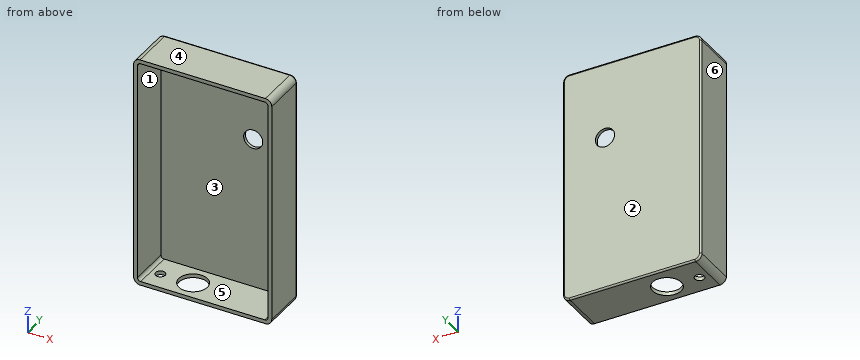
Autodesk Inventor part; units mm, degrees
ref_plane "YZ Plane" through (0, 0, 0) normal (1, 0, 0) x (0, 1, 0)
ref_plane "XZ Plane" through (0, 0, 0) normal (0, 1, 0) x (-1, 0, 0)
ref_plane "XY Plane" through (0, 0, 0) normal (0, 0, 1) x (1, 0, 0)
sketch "Skizze1" plane through (0, 0, 0) normal (0, 1, 0) x (-1, 0, 0)
  line L0 (1, 0) -> (40, 0)
  line L1 (41, 1) -> (41, 70)
  line L2 (40, 71) -> (1, 71)
  line L3 (0, 70) -> (0, 1)
  line L4 (42.2, 70.2) -> (42.2, 0.8)
  line L5 (40.2, -1.2) -> (0.8, -1.2)
  line L6 (-1.2, 0.8) -> (-1.2, 70.2)
  line L7 (0.8, 72.2) -> (40.2, 72.2)
  arc A0 (42.2, 70.2) -> (40.2, 72.2) centre (40.2, 70.2) ccw
  arc A1 (40.2, -1.2) -> (42.2, 0.8) centre (40.2, 0.8) ccw
  arc A2 (-1.2, 0.8) -> (0.8, -1.2) centre (0.8, 0.8) ccw
  arc A3 (0.8, 72.2) -> (-1.2, 70.2) centre (0.8, 70.2) ccw
  arc A4 (41, 70) -> (40, 71) centre (40, 70) ccw
  arc A5 (40, 0) -> (41, 1) centre (40, 1) ccw
  arc A6 (0, 1) -> (1, 0) centre (1, 1) ccw
  arc A7 (1, 71) -> (0, 70) centre (1, 70) ccw
  point P0 (0, 0)
  point P1 (41, 71)
  point P2 (41, 0)
  point P3 (0, 71)
  dimension "d0" = 41
  dimension "d1" = 71
  dimension "d2" = 1.2
  dimension "d3" = 2
  dimension "d4" = 1
extrude "Extrusion1" add sketch "Skizze1" along normal blind 13
sketch "Skizze2" plane through (0, 13, 0) normal (0, 1, 0) x (1, 0, 0)
  line L0 (1.2, -70.2) -> (1.2, -0.8)
  arc A0 (1.2, -0.8) -> (-0.8, 1.2) centre (-0.8, -0.8) ccw
  line L1 (-0.8, 1.2) -> (-40.2, 1.2)
  arc A1 (-40.2, 1.2) -> (-42.2, -0.8) centre (-40.2, -0.8) ccw
  line L2 (-42.2, -0.8) -> (-42.2, -70.2)
  arc A2 (-42.2, -70.2) -> (-40.2, -72.2) centre (-40.2, -70.2) ccw
  line L3 (-40.2, -72.2) -> (-0.8, -72.2)
  arc A3 (-0.8, -72.2) -> (1.2, -70.2) centre (-0.8, -70.2) ccw
  arc A4 (0, -1) -> (-1, 0) centre (-1, -1) ccw
  line L4 (0, -1) -> (0, -70)
  arc A5 (-1, -71) -> (0, -70) centre (-1, -70) ccw
  line L5 (-1, -71) -> (-40, -71)
  arc A6 (-41, -70) -> (-40, -71) centre (-40, -70) ccw
  line L6 (-41, -70) -> (-41, -1)
  arc A7 (-40, 0) -> (-41, -1) centre (-40, -1) ccw
  line L7 (-40, 0) -> (-1, 0)
  point P0 (0, 0)
extrude "Extrusion2" add sketch "Skizze2" along normal blind 1 contours A3 L3 A2 L2 A1 L1 A0 L0 | L4 A5 L5 A6 L6 A7 L7 A4
fillet "Rundung1" radius 0.5 8 edges at (0.6142, 14, -0.6142) (-20.5, 14, -1.2) (-41.6142, 14, -0.6142) (-42.2, 14, 35.5) (-41.6142, 14, 71.6142) (-20.5, 14, 72.2) (0.6142, 14, 71.6142) (1.2, 14, 35.5)
sketch "Skizze3" plane through (0, 14, 0) normal (0, 1, 0) x (1, 0, 0)
  circle A0 centre (-12, -48) radius 3
  line L0 (0, -1) -> (0, -70)
  line L1 (-40, 0) -> (-1, 0)
  point P0 (0, 0)
  dimension "d10" = 6
  dimension "d11" = 12
  dimension "d12" = 48
extrude "Extrusion3" cut sketch "Skizze3" against normal blind 1
sketch "Skizze4" plane through (-0.8, 0, -1.2) normal (0, 0, -1) x (-1, 0, 0)
  circle A0 centre (26.4, 6.5) radius 4.5
  line L0 (0, 0) -> (39.4, 0)
  line L1 (41.4, 0) -> (41.4, 13.5)
  circle A1 centre (36.4, 6) radius 1.5
  point P0 (-0.8, 0)
  dimension "d15" = 9
  dimension "d16" = 6.5
  dimension "d17" = 15
  dimension "d18" = 3
  dimension "d19" = 5
extrude "Extrusion4" cut sketch "Skizze4" against normal blind 5
properties part number "wanne"
The listing builds one solid part. Answer for the finished solid, in the listing's coordinates (mm). Face numbers are marked on the shaded views. A direction names the side the tool comes from. Round coordinates to 2 decimals unless told otherwise and drop trailing zeros. Write each loop counter-clockwise with the first axis right and the second up, starting at its lowest first coordinate (ties: lowest second). Pieces come first, ordered by that corner, then holes. Notation, with made-up numbers: (48, 89) - (93, 89) arc R23 cw to (93, 100) - close; hole circle Ø11 at (14, 67.5). An arc over 180 degrees is marked (long way). Use a Markdown table: item, result. Add a question column.
1. A tool of negligible diameter and unlimited length cuts with its end or side. For the marked faces 1 and 2, from which of +Z, -Z, +X, -X, +Y, -Y can it reach the whole face along a straight path? Write none if from no direction.
2. The part is cut by section B-B (z = 57.5). Write down the section's boundary in (x, y), and give its area (3 significant figures).
3. Flat-ended cylindrical pins translate along their axes: P1, Ø5.5, axis at x = -27.2, y = 6.5, coming from the -Z side; P2, Ø20.5, axis at x = -30, z = 29.5, coming from the -Y side; P3, Ø4, axis at x = -37.2, y = 6, coming from the -Z side. Find the tip coordinate at first contact, or state that the pin passes through.
4. The part is cut by section A-A (x = -12). Write down the section's boundary in (y, z), and give its area (3 significant figures).
5. Consider line 1 (X direction, y = 9.5, z = 43.5); line 2 (Z direction, x = -1, y = 7.25); line 3 (Y direction, x = -37.2, z = -0.55). Determine where each line is inside the solid, lowest interval first.
6. For a pull along Z with two mould halves and no side action, classify the marked faces 3, 4, 5 and 6 as +Z half, -Z half, draft (parallel to the pull), parting line (faces both ways), or undercut.
7. The part is cut by section D-D (y = 5.25). Write down the section's boundary in (x, z), and give its area (3 significant figures).
8. The part is cut by section C-C (x = -18). Write down the section's boundary in (y, z), and give its area (3 significant figures).
Reported:
| question | item | result |
|---|---|---|
| 1 | face 1 | -Y |
| 1 | face 2 | +Z, -Z, +X, -X, +Y |
| 2 | outline | (-42.2, 0) - (-41, 0) - (-41, 13) - (0, 13) - (0, 0) - (1.2, 0) - (1.2, 13.5) arc R0.5 ccw to (0.7, 14) - (-41.7, 14) arc R0.5 ccw to (-42.2, 13.5) - close |
| 2 | area | 74.5 mm^2 |
| 3 | P1 | z = 71 |
| 3 | P2 | y = 13 |
| 3 | P3 | z = -1.2 |
| 4 | outline | (0, -1.2) - (13.5, -1.2) arc R0.5 ccw to (14, -0.7) - (14, 45) - (13, 45) - (13, 0) - (0, 0) - close; (0, 71) - (13, 71) - (13, 51) - (14, 51) - (14, 71.7) arc R0.5 ccw to (13.5, 72.2) - (0, 72.2) - close |
| 4 | area | 98.5 mm^2 |
| 5 | line 1 | -42.2 to -41, 0 to 1.2 |
| 5 | line 2 | -1.2 to 0, 71 to 72.2 |
| 5 | line 3 | 0 to 4.5, 7.5 to 14 |
| 6 | face 3 | undercut |
| 6 | face 4 | +Z half |
| 6 | face 5 | undercut |
| 6 | face 6 | draft |
| 7 | outline | (-42.2, 0.8) arc R2 ccw to (-40.2, -1.2) - (-38.5, -1.2) - (-38.5, 0) - (-40, 0) arc R1 cw to (-41, 1) - (-41, 70) arc R1 cw to (-40, 71) - (-1, 71) arc R1 cw to (0, 70) - (0, 1) arc R1 cw to (-1, 0) - (-22.88, 0) - (-22.88, -1.2) - (-0.8, -1.2) arc R2 ccw to (1.2, 0.8) - (1.2, 70.2) arc R2 ccw to (-0.8, 72.2) - (-40.2, 72.2) arc R2 ccw to (-42.2, 70.2) - close; (-35.9, -1.2) - (-31.52, -1.2) - (-31.52, 0) - (-35.9, 0) - close |
| 7 | area | 258 mm^2 |
| 8 | outline | (0, -1.2) - (13.5, -1.2) arc R0.5 ccw to (14, -0.7) - (14, 71.7) arc R0.5 ccw to (13.5, 72.2) - (0, 72.2) - (0, 71) - (13, 71) - (13, 0) - (0, 0) - close |
| 8 | area | 104 mm^2 |
